Can you work these out from the model? Positions are in its coordinate system, mm. Face numbers are marked on the shaded views. A direction names the side the tool comes from. Round coordinates to 2 decimals unless told otherwise and drop trailing zeros. Write each loop counter-clockwise with the first axis right and the second up, starting at its lowest first coordinate (ties: lowest second). Pieces come first, ordered by that corner, then holes. Notation, with made-up numbers: (-3.75, 72.25) -> (11.25, 72.25) arc R16 cw to (11.25, 89.25) -> close; hole circle Ø6 at (77.5, 50.25). An arc over 180 degrees is marked (long way). Use CSV: the item, a comma, the result in double quotes.
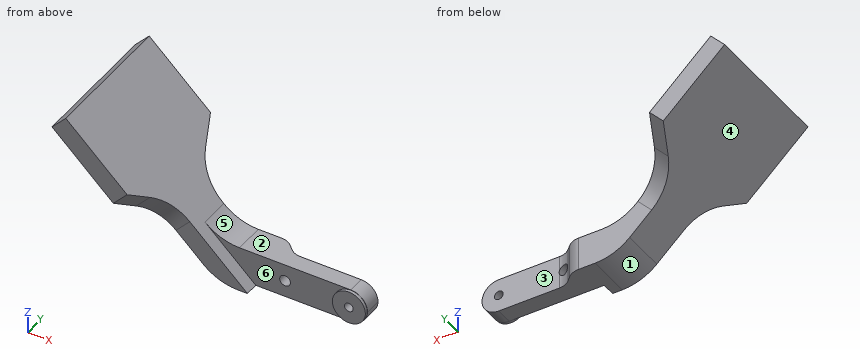
```python
from build123d import *

# Parameters (mm, degrees)
BOSS_EXTRUDE1_DEPTH = 5
FILLET1_R           = 5
SKETCH2_R           = 1.2999999999999945
CUT_EXTRUDE1_DEPTH  = 10
BOSS_EXTRUDE2_DEPTH = 20
BOSS_EXTRUDE3_DEPTH = 15
BOSS_EXTRUDE4_DEPTH = 6
SKETCH6_R           = 4.900000000000002
SKETCH6_R_2         = 1.299999999999994
BOSS_EXTRUDE5_DEPTH = 0.9
BOSS_EXTRUDE6_DEPTH = 3.9999999999999964
BOSS_EXTRUDE7_DEPTH = 3.9999999999999964
FILLET2_R           = 15
FILLET7_SIZE        = 5
FILLET8_R           = 5
SKETCH10_R          = 1.6000000000000019
CUT_EXTRUDE2_DEPTH  = 10


# Some blends are built 0.0001 mm under size
with BuildPart() as part:
    # Sketch1 → Boss-Extrude1 (new body)
    with BuildSketch(Plane(origin=(0, 0, 0), x_dir=(1, 0, 0), z_dir=(0, 1, 0))):
        Polygon((4.091990160374978, 5.611877790284978), (0, 10), (0, 1.79603523340848), align=None)
        Polygon((0, 1.79603523340848), (0, 10), (-42.4185146939121, -29.55590488362469), (-38.32652453353713, -33.94402709333974), (-1.9260119864091507, 0), align=None)
        Polygon((42, 10), (0, 10), (4.091990160374978, 5.611877790284978), (0, 1.7960352334084817), (0, 0), (42, 0), align=None)
        Polygon((0, 0), (0, 1.79603523340848), (-1.9260119864091507, 0), align=None)
    extrude(amount=BOSS_EXTRUDE1_DEPTH)

    # Fillet1
    fillet1_edges = [part.edges().sort_by_distance(p)[0] for p in [
        (42, 2.5, 0),
        (42, 2.5, -10),
    ]]
    fillet(fillet1_edges, radius=FILLET1_R - 0.0001)  # a hair under: the kernel refuses the full size

    # Sketch2 → Cut-Extrude1 (cut)
    with BuildSketch(Plane(origin=(0, 5, 0), x_dir=(1, 0, 0), z_dir=(0, 1, 0))):
        with Locations(Location((37.00000000000001, 4.999999999999989, 0), (0, 0, 270))):
            Circle(SKETCH2_R)
    extrude(amount=-CUT_EXTRUDE1_DEPTH, mode=Mode.SUBTRACT)

    # Sketch3 → Boss-Extrude2 (add)
    with BuildSketch(Plane(origin=(0, 5, 0), x_dir=(1, 0, 0), z_dir=(0, 1, 0))):
        Polygon((-42.4185146939121, -29.55590488362471), (-38.32652453353713, -33.94402709333974), (-20.126268259973138, -16.97201354666987), (-24.21825842034811, -12.583891336954824), align=None)
    extrude(amount=BOSS_EXTRUDE2_DEPTH)

    # Sketch4 → Boss-Extrude3 (add)
    with BuildSketch(Plane.XZ):
        Polygon((-42.4185146939121, 29.55590488362471), (-38.32652453353713, 33.94402709333974), (-20.126268259973134, 16.972013546669885), (-24.218258420348107, 12.583891336954828), align=None)
    extrude(amount=BOSS_EXTRUDE3_DEPTH)

    # Sketch5 → Boss-Extrude4 (add)
    with BuildSketch(Plane(origin=(-4.987820251299118, 0, -5.348782368720677), x_dir=(-0.7313537016191739, 0, 0.6819983600624947), z_dir=(-0.6819983600624948, 0, -0.731353701619174))):
        Polygon((26.29430619749914, -15), (26.29430619749914, 0), (13.888976828400956, 0), align=None)
        Polygon((13.888976828400958, 5), (26.29430619749914, 25), (26.29430619749914, 5), align=None)
    extrude(amount=-BOSS_EXTRUDE4_DEPTH)

    # Sketch6 → Boss-Extrude5 (add)
    with BuildSketch(Plane.XZ):
        with Locations(Location((37.00000000000001, -4.999999999999989, 0), (0, 0, 90))):
            Circle(SKETCH6_R)
        with Locations(Location((37.00000000000001, -4.999999999999989, 0), (0, 0, 90))):
            Circle(SKETCH6_R_2, mode=Mode.SUBTRACT)
    extrude(amount=BOSS_EXTRUDE5_DEPTH)

    # Sketch8 → Boss-Extrude6 (add)
    with BuildSketch(Plane.XZ):
        Polygon((0, -10), (-19.681916643400598, 8.353684194074795), (-15.589926483025625, 12.741806403789838), (8.797675113837775, -10), align=None)
    extrude(amount=BOSS_EXTRUDE6_DEPTH)

    # Sketch9 → Boss-Extrude7 (add)
    with BuildSketch(Plane(origin=(0, 5, 0), x_dir=(1, 0, 0), z_dir=(0, 1, 0))):
        Polygon((0, 10), (-20.891607783919927, -9.48173943217613), (-16.79961762354496, -13.869861641891177), (-1.92601198640914, -7.11e-15), (17.950520425486616, 5.22e-15), (17.950520425486616, 10), align=None)
    extrude(amount=BOSS_EXTRUDE7_DEPTH)

    # Fillet2
    fillet2_edges = [part.edges().sort_by_distance(p)[0] for p in [
        (-14.914116497044613, 8.999999999999996, 8.009621013204299),
        (-1.9260119864091478, 4.499999999999998, 2.06e-15),
        (0, 2.5, -10),
        (-15.518962067304274, -3.9999999999999973, 8.573648632254974),
    ]]
    fillet(fillet2_edges, radius=FILLET2_R)

    # Fillet7
    # the kernel refuses this chamfer: 5 mm, written as the material it takes off along each edge
    with BuildSketch(Plane(origin=(17.950520425486616, 8.999999999999996, 12.858414939829549), x_dir=(0.027495876610586317, -0.9996219169112968, 0), z_dir=(0, 0, -1))) as fillet7_piece_1_section:
        Polygon((FILLET7_SIZE * 0.999621916911, FILLET7_SIZE * 0.0274958766106), (-FILLET7_SIZE * 0.0274958766106, FILLET7_SIZE * 0.999621916911), (0, 0), align=None)
    fillet7_piece_1 = extrude(amount=35.71682987965911, mode=Mode.PRIVATE)
    fillet7_piece_1 = split(fillet7_piece_1, bisect_by=Plane(origin=(16.221928363932022, 5, -5.000000000000004), z_dir=(0, 1, 0)), keep=Keep.TOP, mode=Mode.PRIVATE)
    add(fillet7_piece_1, mode=Mode.SUBTRACT)

    # Fillet8
    fillet8_edges = [part.edges().sort_by_distance(p)[0] for p in [
        (12.95052042548848, 8.999999999998002, -5.000000000000002),
        (16.950520425489678, 5, -4.999999999999999),
    ]]
    fillet(fillet8_edges, radius=FILLET8_R)

    # Sketch10 → Cut-Extrude2 (cut)
    with BuildSketch(Plane(origin=(0, 0, 0), x_dir=(-1, 0, 0), z_dir=(0, -1, 0))):
        with Locations(Location((-17.499999999999247, 5.000000000001407, 0), (0, 0, 90))):
            Circle(SKETCH10_R)
    extrude(amount=-CUT_EXTRUDE2_DEPTH, mode=Mode.SUBTRACT)


solid = part.part
```
Q1. Suppose I cut it at C-C (x = 27). Write out the boundary of the cut face in (y, z).
Resolved:
outline,"(0, -10) -> (5, -10) -> (5, 0) -> (0, 0) -> close"
Q2. Suppose I cut it at A-A (y = 4). Count the separate pieces of the cut face and the enclosed holes in it, and give its area (3 significant figures).
Resolved:
separate pieces,"1"
enclosed holes,"2"
area,"729 mm^2"
Q3. Suppose I cut it at B-B (x = 17.5). Write out the boundary of the cut face in (y, z), and give its area (3 significant figures).
Resolved:
outline,"(0, -10) -> (5.24, -10) -> (5.24, -6.6) -> (0, -6.6) -> close; (0, -3.4) -> (5.24, -3.4) -> (5.24, 0) -> (0, 0) -> close"
area,"35.6 mm^2"
Q4. Suppose I cut it at D-D (z = -2.5). Write out the boundary of the cut face in (x, y).
Resolved:
outline,"(-8.04, -4) -> (0.75, -4) -> (0.75, 0) -> (32.79, 0) -> (32.79, -0.9) -> (41.21, -0.9) -> (41.21, 0) -> (41.33, 0) -> (41.33, 5) -> (19.02, 5) arc R5 cw to (15.49, 6.46) -> (14.41, 7.54) arc R5 ccw to (10.88, 9) -> (-8.04, 9) -> close"
Q5. Please list where these lines run through material, in increasing order: probe 1 along Z at (x, y) = (17.5, 4.25); probe 2 along X at (y, z) = (0.55, -5); probe 3 along Y at (x, z) = (-11, 0.5).
Resolved:
probe 1,"z = -10 to -6.6, -3.4 to 0"
probe 2,"x = -5.36 to 15.9, 19.1 to 35.7, 38.3 to 42"
probe 3,"y = -4 to 9"
Q6. If we mould it in two halves opening along X, with no side actions, what happens to the marked faces 3, 4, 5 and 6? For each: released by +X, released by -X, zero draft, split by the parting line, or undercut.
Resolved:
face 3,"zero draft"
face 4,"released by -X"
face 5,"released by +X"
face 6,"undercut"
Q7. On a 3-axis mill with a long thin cutter (end or side, diameter ignored), from which of +Z, -Z, +X, -X, +Y, -Y can I reach the whole of each face in a straight line? I mean the marked faces 1 and 2. Say none if no direction works.
Resolved:
face 1,"-Z, -X, +Y, -Y"
face 2,"+Z, +X, +Y, -Y"
Q8. Will these pins go through, and if not, where does the flat tip stop? P1, Ø2.5, axis at x = 17.5, z = -5, coming from the +Y side; P2, Ø6, axis at x = -5.5, y = -5, coming from the +Z side; P3, Ø3, axis at x = 35.5, z = -6, coming from the +Y side; P4, Ø8, axis at x = 1, z = 1.5, coming from the -Y side.
Resolved:
P1,"passes through"
P2,"stops at z = 5.97"
P3,"stops at y = 5"
P4,"stops at y = -4"
